Read the model definition and answer for the solid it produces. Units are mm, in the model's axes. A direction names the side the tool comes from. Round coordinates to 2 decimals unless told otherwise and drop trailing zeros. Write each loop counter-clockwise with the first axis right and the second up, starting at its lowest first coordinate (ties: lowest second). Pieces come first, ordered by that corner, then holes. Notation, with made-up numbers: (3, 66) -> (31, 66) arc R33 cw to (31, 97) -> close; hole circle Ø11 at (41.25, -31.75). An arc over 180 degrees is marked (long way). Return JSON: item names as keys, results as strings.
from build123d import *

# Parameters (mm, degrees)
EXTRUDE_1_DEPTH   = 2.5
EXTRUDE_1_2_DEPTH = 2.5
SKETCH_1_7_W      = 40
SKETCH_1_7_H      = 20
EXTRUDE_4_DEPTH   = 27
SKETCH_1_8_W      = 40
SKETCH_1_8_H      = 20
EXTRUDE_5_DEPTH   = 11.5
EXTRUDE_6_DEPTH   = 5.5
SKETCH_2_3_R      = 6.75
SKETCH_2_3_R_2    = 3
EXTRUDE_7_DEPTH   = 1.5


with BuildPart() as part:
    # Sketch 1 → Extrude 1 (new body)
    with BuildSketch(Plane(origin=(0, 0, 0), x_dir=(1, 0, 0), z_dir=(0, 1, 0))):
        with BuildLine():
            Line((-20, -8.75), (-20, 8.75))
            Line((-20, 8.75), (-26.75, 8.75))
            Line((-26.75, 8.75), (-26.75, 6.25))
            Line((-26.75, 6.25), (-25.0612495, 6.25))
            ThreePointArc((-25.0612495, 6.25), (-22.837617557, 6.887127314), (-21.5, 5))
            ThreePointArc((-21.5, 5), (-22.837617557, 3.112872686), (-25.0612495, 3.75))
            Line((-25.0612495, 3.75), (-26.75, 3.75))
            Line((-26.75, 3.75), (-26.75, -3.75))
            Line((-26.75, -3.75), (-25.0612495, -3.75))
            ThreePointArc((-25.0612495, -3.75), (-22.837617557, -3.112872686), (-21.5, -5))
            ThreePointArc((-21.5, -5), (-22.837617557, -6.887127314), (-25.0612495, -6.25))
            Line((-25.0612495, -6.25), (-26.75, -6.25))
            Line((-26.75, -6.25), (-26.75, -8.75))
            Line((-26.75, -8.75), (-20, -8.75))
        make_face()
    extrude(amount=EXTRUDE_1_DEPTH)



with BuildPart() as body_2:
    # Sketch 1 → Extrude 1 2 (new body)
    with BuildSketch(Plane(origin=(0, 0, 0), x_dir=(1, 0, 0), z_dir=(0, 1, 0))):
        with BuildLine():
            Line((26.75, 8.75), (20, 8.75))
            Line((20, 8.75), (20, -8.75))
            Line((20, -8.75), (26.75, -8.75))
            Line((26.75, -8.75), (26.75, -6.25))
            Line((26.75, -6.25), (25.0612495, -6.25))
            ThreePointArc((25.0612495, -6.25), (21.5, -5), (25.0612495, -3.75))
            Line((25.0612495, -3.75), (26.75, -3.75))
            Line((26.75, -3.75), (26.75, 3.75))
            Line((26.75, 3.75), (25.0612495, 3.75))
            ThreePointArc((25.0612495, 3.75), (21.5, 5), (25.0612495, 6.25))
            Line((25.0612495, 6.25), (26.75, 6.25))
            Line((26.75, 6.25), (26.75, 8.75))
        make_face()
    extrude(amount=EXTRUDE_1_2_DEPTH)


with BuildPart() as body_3:
    # Sketch 1_7 → Extrude 4 (new body)
    with BuildSketch(Plane(origin=(0, 0, 0), x_dir=(1, 0, 0), z_dir=(0, 1, 0))):
        Rectangle(SKETCH_1_7_W, SKETCH_1_7_H)
    extrude(amount=-EXTRUDE_4_DEPTH)


with BuildPart() as part_1:
    add(part.part)

    add(body_2.part)  # Extrude 5 merges body 2

    add(body_3.part)  # Extrude 5 merges body 3
    # Sketch 1_8 → Extrude 5 (add)
    with BuildSketch(Plane(origin=(0, 0, 0), x_dir=(1, 0, 0), z_dir=(0, 1, 0))):
        Rectangle(SKETCH_1_8_W, SKETCH_1_8_H)
    extrude(amount=EXTRUDE_5_DEPTH)

    # Sketch 2 → Extrude 6 (add)
    with BuildSketch(Plane(origin=(0, 11.5, 0), x_dir=(1, 0, 0), z_dir=(0, 1, 0))):
        with BuildLine():
            ThreePointArc((7, 0), (10, -3), (13, 0))
            Line((13, 0), (7, 0))
        make_face()
        with BuildLine():
            Line((7, 0), (13, 0))
            ThreePointArc((13, 0), (10, 3), (7, 0))
        make_face()
    extrude(amount=EXTRUDE_6_DEPTH)

    # Sketch 2_3 → Extrude 7 (add)
    with BuildSketch(Plane(origin=(0, 11.5, 0), x_dir=(1, 0, 0), z_dir=(0, 1, 0))):
        with Locations(Location((10, 0, 0), (0, 0, 270))):
            Circle(SKETCH_2_3_R)
        with Locations(Location((10, 0, 0), (0, 0, 270))):
            Circle(SKETCH_2_3_R_2, mode=Mode.SUBTRACT)
    extrude(amount=EXTRUDE_7_DEPTH)


solid = part_1.part
Item 1: Straight lines are drawn through the part: L1, parallel to Z at x = 23.5, y = 1.45; L2, parallel to Y at x = 16, z = -5.25; L3, parallel to Z at x = 24.5, y = 1. For each, find the intervals that lie inside material, in ascending order. Write a range as [from, to].
Worked answers:
{"L1": "z = [-8.75, -7], [-3, 3], [7, 8.75]", "L2": "y = [-27, 11.5]", "L3": "z = [-8.75, -6.73], [-3.27, 3.27], [6.73, 8.75]"}
Item 2: Section B-B (z = 0) is taken. Give the vertices of the cut face in (x, y), then the cut area to 3 significant figures.
Worked answers:
{"outline": "(-26.75, 0) -> (-20, 0) -> (-20, -27) -> (20, -27) -> (20, 0) -> (26.75, 0) -> (26.75, 2.5) -> (20, 2.5) -> (20, 11.5) -> (16.75, 11.5) -> (16.75, 13) -> (13, 13) -> (13, 17) -> (7, 17) -> (7, 13) -> (3.25, 13) -> (3.25, 11.5) -> (-20, 11.5) -> (-20, 2.5) -> (-26.75, 2.5) -> close", "area": "1,620 mm2"}
Item 3: A tool of negligible diameter and unlimited length cuts with its end or side. For faces 1 (the flat face through (23, 1, 8.75)), 2 (the cylindrical face through (12.86, 14.97, -0.9)), 3 (the flat face through (23, 0, 0)), from which of +Z, -Z, +X, -X, +Y, -Y can it reach the whole face along a straight path? Write none if from no direction.
Worked answers:
{"face 1": "+Z, +X, +Y, -Y", "face 2": "+Y", "face 3": "+Z, -Z, +X, -Y"}
Item 4: For a pull along Z with two mould halves and no side action, classify faces 4 (the cylindrical face through (21.5, 1.23, -4.93)), 5 (the flat face through (0, -8, 10)), 6 (the flat face through (20, -8, 0)) as released by +Z, released by -Z, zero draft, split by the parting line, or undercut.
Worked answers:
{"face 4": "undercut", "face 5": "released by +Z", "face 6": "zero draft"}
Item 5: Section D-D (y = 4) is taken. Give the vertices of the cut face in (x, z).
Worked answers:
{"outline": "(-20, -10) -> (20, -10) -> (20, 10) -> (-20, 10) -> close"}
Item 6: Flat-ended cylindrical pins translate along their axes: pin 1 (5.5 mm diameter, centred on x = -22.5, z = 2, fed in from +Y); pin 2 (1.4 mm diameter, centred on x = -26, y = 1, fed in from -Z); pin 3 (1.9 mm diameter, centred on x = -25.5, y = 1.5, fed in from +Z). Find the tip coordinate at first contact, or state that the pin passes through.
Worked answers:
{"pin 1": "stops at y = 11.5", "pin 2": "stops at z = -8.75", "pin 3": "stops at z = 8.75"}
Item 7: Section C-C (x = 10) is taken. Give the vertices of the cut face in (y, z).
Worked answers:
{"outline": "(-27, -10) -> (11.5, -10) -> (11.5, -6.75) -> (13, -6.75) -> (13, -3) -> (17, -3) -> (17, 3) -> (13, 3) -> (13, 6.75) -> (11.5, 6.75) -> (11.5, 10) -> (-27, 10) -> close"}
Item 8: Section A-A (x = 23.5) is taken. Give the vertices of the cut face in (y, z).
Worked answers:
{"outline": "(0, -8.75) -> (2.5, -8.75) -> (2.5, -7) -> (0, -7) -> close; (0, -3) -> (2.5, -3) -> (2.5, 3) -> (0, 3) -> close; (0, 7) -> (2.5, 7) -> (2.5, 8.75) -> (0, 8.75) -> close"}
